```python
from build123d import *

# Parameters (mm, degrees)
BOX105_W     = 140
BOX105_H     = 80
BOX105_DEPTH = 180
BOX104_W     = 140
BOX104_H     = 80
BOX104_DEPTH = 180
BOX106_W     = 390
BOX106_H     = 140
BOX106_DEPTH = 190


with BuildPart() as cube077:
    # Box105 → Box105 (new body)
    with BuildSketch(Plane(origin=(220, 30, 0), x_dir=(1, 0, 0), z_dir=(0, 0, 1))):
        with Locations((70, 40)):
            Rectangle(BOX105_W, BOX105_H)
    extrude(amount=BOX105_DEPTH)


with BuildPart() as fusion018:
    # Box104 → Box104 (new body)
    with BuildSketch(Plane(origin=(30, 30, 0), x_dir=(1, 0, 0), z_dir=(0, 0, 1))):
        with Locations((70, 40)):
            Rectangle(BOX104_W, BOX104_H)
    extrude(amount=BOX104_DEPTH)

    # Fusion018: union Cube077
    add(cube077.part)


with BuildPart() as cut013:
    # Box106 → Box106 (new body)
    with BuildSketch(Plane.XY):
        with Locations((195, 70)):
            Rectangle(BOX106_W, BOX106_H)
    extrude(amount=BOX106_DEPTH)

    # Cut013: cut Fusion018
    add(fusion018.part, mode=Mode.SUBTRACT)


with BuildPart() as cut013_1:
    # Cut013 placement: moved
    add(cut013.part.moved(Location((340, 445, -190))))


solid = cut013_1.part
```
Geometry: final body of the model. Coordinates: model frame, mm. A direction names the side the tool comes from. Coordinates: 2 decimals unless noted, no trailing zeros. Order: outer loops, then holes, each group sorted by start corner. A loop starts at its lowest first (then second) coordinate and runs counter-clockwise, first axis right, second up. Notation, with made-up numbers: (-31, -31.75) -> (-2, -31.75) arc R19 ccw to (-2, -8.75) -> close; hole circle Ø3 at (-3, 33). An arc over 180 degrees is marked (long way). Write item = value, one per line.
(1) Line query: line 1 (X direction, y = 538, z = -70); line 2 (Y direction, x = 398.5, z = -140); line 3 (Z direction, x = 485.5, y = 544.5). Output: solid intervals per line, ascending.
Solved:
line_1 = 340 to 370, 510 to 560, 700 to 730
line_2 = 445 to 475, 555 to 585
line_3 = -10 to 0
(2) Pin query (flat end, axial travel): pin 1 Ø24 at (x, y) = (454, 511.5) entering from -Z. Return the tip coordinate at first contact, or that it passes through.
Solved:
pin_1 = -10
(3) Access query for faces 5 (the flat face through (532, 516, -190)), 6 (the flat face through (700, 514, -101)). Directions: +Z, -Z, +X, -X, +Y, -Y. A direction counts if a zero-diameter tool reaches every point of the face in a straight line with its end or side. Return the directions, or none.
Solved:
face_5 = -Z, +X, -X, +Y, -Y
face_6 = -Z
(4) Pull-direction query (Y, two-part tool) for faces 1 (the flat face through (629, 516, -10)), 2 (the flat face through (340, 514, -96)), 3 (the flat face through (560, 514, -101)), 4 (the flat face through (532, 445, -96)); classes: pulls with the +Y half, pulls with the -Y half, needs draft (parallel to the pull), parting line crosses it, or undercut.
Solved:
face_1 = undercut
face_2 = needs draft
face_3 = undercut
face_4 = pulls with the -Y half
(5) Cut plane B-B on x = 407.5. Return loops of the section in (y, z).
Solved:
outline = (445, -190) -> (475, -190) -> (475, -10) -> (555, -10) -> (555, -190) -> (585, -190) -> (585, 0) -> (445, 0) -> close
(6) Cut plane A-A on z = -101. Return loops of the section in (x, y).
Solved:
outline = (340, 445) -> (730, 445) -> (730, 585) -> (340, 585) -> close; hole (370, 475) -> (510, 475) -> (510, 555) -> (370, 555) -> close; hole (560, 475) -> (700, 475) -> (700, 555) -> (560, 555) -> close
(7) Cut plane C-C on y = 551. Return loops of the section in (x, z).
Solved:
outline = (340, -190) -> (370, -190) -> (370, -10) -> (510, -10) -> (510, -190) -> (560, -190) -> (560, -10) -> (700, -10) -> (700, -190) -> (730, -190) -> (730, 0) -> (340, 0) -> close
